```python
from build123d import *

# Parameters (mm, degrees)
SKETCH_1_W               = 80
SKETCH_1_H               = 30
EXTRUDE_1_DEPTH          = 8
CUT_EXTRUDE_1_DEPTH      = 9
SKETCH_3_W               = 2.4
SKETCH_3_H               = 9
CUT_EXTRUDE_2_DEPTH      = 1
CUT_EXTRUDE_2_DEPTH_BACK = 9
SKETCH_5_R               = 1.5
CUT_EXTRUDE_3_DEPTH      = 32
SKETCH_6_W               = 3
SKETCH_6_H               = 8
CUT_EXTRUDE_5_DEPTH      = 5
SKETCH_7_R               = 1.5
CUT_EXTRUDE_6_DEPTH      = 32


with BuildPart() as part:
    # 草图1 → 凸台-拉伸1 (new body)
    with BuildSketch(Plane(origin=(0, 0, 0), x_dir=(1, 0, 0), z_dir=(0, 1, 0))):
        Rectangle(SKETCH_1_W, SKETCH_1_H)
    extrude(amount=EXTRUDE_1_DEPTH)

    # 草图2 → 切除-拉伸1 (cut, through all)
    with BuildSketch(Plane(origin=(0, 8, 0), x_dir=(1, 0, 0), z_dir=(0, 1, 0))):
        with BuildLine():
            Line((-24.5, 3), (-24.5, -15))
            Line((-24.5, -15), (-23.5, -15))
            Line((-23.5, -15), (-23.5, 0.763932023))
            ThreePointArc((-23.5, 0.763932023), (-18.761387212, 4.224744871), (-24.5, 3))
        make_face()
        with BuildLine():
            Line((23.5, -15), (23.5, 0.763932023))
            ThreePointArc((23.5, 0.763932023), (18.761387212, 4.224744871), (24.5, 3))
            Line((24.5, 3), (24.5, -15))
            Line((24.5, -15), (23.5, -15))
        make_face()
    extrude(amount=-CUT_EXTRUDE_1_DEPTH, mode=Mode.SUBTRACT)

    # 草图3 → 切除-拉伸2 (cut, two sides)
    with BuildSketch(Plane(origin=(0, 8, 0), x_dir=(1, 0, 0), z_dir=(0, 1, 0))) as cut_extrude_2_sk:
        with Locations((-5.7, -10.5)):
            Rectangle(SKETCH_3_W, SKETCH_3_H)
        with Locations((5.7, -10.5)):
            Rectangle(SKETCH_3_W, SKETCH_3_H)
    extrude(amount=CUT_EXTRUDE_2_DEPTH, mode=Mode.SUBTRACT)
    extrude(cut_extrude_2_sk.sketch, amount=-CUT_EXTRUDE_2_DEPTH_BACK, mode=Mode.SUBTRACT)

    # 草图5 → 切除-拉伸3 (cut)
    with BuildSketch(Plane.ZY.offset(40)):
        with Locations((12, 4)):
            Circle(SKETCH_5_R)
    extrude(amount=-CUT_EXTRUDE_3_DEPTH, mode=Mode.SUBTRACT)

    # 草图6 → 切除-拉伸5 (cut)
    with BuildSketch(Plane.XY.offset(15)):
        with Locations((-17, 4)):
            Rectangle(SKETCH_6_W, SKETCH_6_H)
        with Locations((17, 4)):
            Rectangle(SKETCH_6_W, SKETCH_6_H)
    extrude(amount=-CUT_EXTRUDE_5_DEPTH, mode=Mode.SUBTRACT)

    # 草图7 → 切除-拉伸6 (cut)
    with BuildSketch(Plane(origin=(40, 0, 0), x_dir=(0, 0, -1), z_dir=(1, 0, 0))):
        with Locations((-12, 4)):
            Circle(SKETCH_7_R)
    extrude(amount=-CUT_EXTRUDE_6_DEPTH, mode=Mode.SUBTRACT)


solid = part.part
```
Geometry check sheet. Reference: the model listing, model coordinates, mm. A direction names the side the tool comes from. Give positions to 0.01 mm unless a question says otherwise; leave off trailing zeros. Order: outer loops, then holes, each group sorted by start corner. A loop starts at its lowest first (then second) coordinate and runs counter-clockwise, first axis right, second up. Notation, with made-up numbers: (40, -37.5) - (71, -37.5) arc R33 ccw to (71, -8.5) - close; hole circle Ø4 at (36, 51.25). An arc over 180 degrees is marked (long way). Answer in a Markdown table with one row per item. Add a question column.
Q1. Tool access check on faces 1 (the cylindrical face through (-21.04, 4.07, 10.5)), 2 (the flat face through (8, 4, 12)), 3 (the flat face through (24.5, 4, 6)). Record the directions out of +Z, -Z, +X, -X, +Y, -Y that give a thin tool (end or side, any length) a straight path to the whole face; none if there is none.
Q2. Cross-section at A-A, the plane x = 21.5. Enter the section's corners in (y, z).
Q3. Cross-section at C-C, the plane y = 7. Enter the section's corners in (x, z), then the cut area to 3 significant figures.
Q4. Cross-section at B-B, the plane x = -34. Enter the section's corners in (y, z), then the cut area to 3 significant figures.
Q5. Cross-section at D-D, the plane z = -4.25. Enter the section's corners in (x, y), then the cut area to 3 significant figures.
Q6. Material ranges on probe 1 along X at (y, z) = (0.5, 5); probe 2 along X at (y, z) = (3.5, -3); probe 3 along X at (y, z) = (2, 8), recorded low to high. Write a range as from..to.
Q7. Gauge pin test, flat ends, axial feed: pin 1 (2.5 mm diameter, centred on y = 4, z = 12, fed in from -X); pin 2 (2.5 mm diameter, centred on y = 4, z = 12, fed in from +X); pin 3 (2.5 mm diameter, centred on x = 17, y = 5.5, fed in from +Z). Record the tip position at first contact, or that the pin passes through.
Q8. Mould release check, pull along Z, two halves, no side actions. Record for faces 4 (the cylindrical face through (11.8, 4.07, 13.5)), 5 (the flat face through (-6.9, 4, 11)), 6 (the flat face through (11, 4, 15)): pulls with the +Z half, pulls with the -Z half, needs draft (parallel to the pull), parting line crosses it, or undercut.
Check values:
| question | item | result |
|---|---|---|
| 1 | face 1 | -X |
| 1 | face 2 | +X |
| 1 | face 3 | +Z, +Y, -Y |
| 2 | outline | (0, -15) - (8, -15) - (8, -6) - (0, -6) - close; (0, 0) - (8, 0) - (8, 15) - (0, 15) - close; hole circle Ø3 at (4, 12) |
| 3 | outline | (-40, -15) - (40, -15) - (40, 15) - (24.5, 15) - (24.5, -3) arc R3 cw (long way) to (23.5, -0.76) - (23.5, 15) - (18.5, 15) - (18.5, 10) - (15.5, 10) - (15.5, 15) - (6.9, 15) - (6.9, 6) - (4.5, 6) - (4.5, 15) - (-4.5, 15) - (-4.5, 6) - (-6.9, 6) - (-6.9, 15) - (-15.5, 15) - (-15.5, 10) - (-18.5, 10) - (-18.5, 15) - (-23.5, 15) - (-23.5, -0.76) arc R3 cw (long way) to (-24.5, -3) - (-24.5, 15) - (-40, 15) - close |
| 3 | area | 2,240 mm^2 |
| 4 | outline | (0, -15) - (8, -15) - (8, 15) - (0, 15) - close; hole circle Ø3 at (4, 12) |
| 4 | area | 233 mm^2 |
| 5 | outline | (-40, 0) - (-24.23, 0) - (-24.23, 8) - (-40, 8) - close; (-18.77, 0) - (18.77, 0) - (18.77, 8) - (-18.77, 8) - close; (24.23, 0) - (40, 0) - (40, 8) - (24.23, 8) - close |
| 5 | area | 553 mm^2 |
| 6 | probe 1 | x = -40..-24.5, -23.5..23.5, 24.5..40 |
| 6 | probe 2 | x = -40..-24.5, -18.5..18.5, 24.5..40 |
| 6 | probe 3 | x = -40..-24.5, -23.5..-6.9, -4.5..4.5, 6.9..23.5, 24.5..40 |
| 7 | pin 1 | stops at x = -8 |
| 7 | pin 2 | stops at x = 8 |
| 7 | pin 3 | stops at z = 10 |
| 8 | face 4 | undercut |
| 8 | face 5 | needs draft |
| 8 | face 6 | pulls with the +Z half |
